```python
from build123d import *

# Parameters (mm, degrees)
SKETCH1_R            = 49.403
BOSS_EXTRUDE1_DEPTH  = 6.35
THREADED_ROD_HOLES_D = 7.9375
U_BOLT_HOLES_D       = 7.9375


with BuildPart() as part:
    # Sketch1 → Boss-Extrude1 (new body)
    with BuildSketch(Plane(origin=(0, 0, 0), x_dir=(1, 0, 0), z_dir=(0, 1, 0))):
        Circle(SKETCH1_R)
    extrude(amount=BOSS_EXTRUDE1_DEPTH)

    # Threaded Rod Holes (through all)
    with Locations(Plane(origin=(0, 6.35, 0), x_dir=(1, 0, 0), z_dir=(0, 1, 0))):
        with Locations((0, 19.05), (0, -19.05)):
            Hole(THREADED_ROD_HOLES_D / 2)

    # U-Bolt Holes (through all)
    with Locations(Plane(origin=(0, 6.35, 0), x_dir=(1, 0, 0), z_dir=(0, 1, 0))):
        with Locations((-16.66875, 0), (16.66875, 0)):
            Hole(U_BOLT_HOLES_D / 2)


solid = part.part
```
Geometry: final body of the model. Coordinates: model frame, mm. Give positions to 0.01 mm unless a question says otherwise; leave off trailing zeros. Write each loop counter-clockwise with the first axis right and the second up, starting at its lowest first coordinate (ties: lowest second). Pieces come first, ordered by that corner, then holes.
1. Section query D-D, the plane x = 19. Return loops of the section in (y, z).
2. Section query C-C, the plane y = 1.25. Return loops of the section in (x, z), then the cut area to 3 significant figures.
3. Draft query along Z for faces 1 (the cylindrical face through (-39.205, 3.131, 30.061)), 2 (the flat face through (-1, 6.35, -1)), 3 (the cylindrical face through (-20.335, 3.131, 1.52)), 4 (the cylindrical face through (0.517, 3.131, 15.115)). Return one class per face: released by +Z, released by -Z, zero draft, split by the parting line, or undercut.
4. Section query B-B, the plane z = 0. Return loops of the section in (x, y).
5. Line query: probe 1 along Z at (x, y) = (0, 2.5); probe 2 along Z at (x, y) = (1, 4.5); probe 3 along X at (y, z) = (1.75, 19.05). Output: solid intervals per line, ascending.
6. Pin query (flat end, axial travel): P1, Ø3, axis at y = 2.5, z = -0.5, coming from the -X side; P2, Ø2, axis at y = 2, z = 30, coming from the +X side. Return the tip coordinate at first contact, or that it passes through.
7. Section query A-A, the plane x = 0. Return loops of the section in (y, z), then the cut area to 3 significant figures.
Computed:
1. outline: (0, -45.6) - (6.35, -45.6) - (6.35, -3.21) - (0, -3.21) - close; (0, 3.21) - (6.35, 3.21) - (6.35, 45.6) - (0, 45.6) - close
2. outline: circle Ø98.81 at (0, 0); hole circle Ø7.94 at (-16.67, 0); hole circle Ø7.94 at (0, -19.05); hole circle Ø7.94 at (0, 19.05); hole circle Ø7.94 at (16.67, 0)
2. area: 7,470 mm2
3. face 1: split by the parting line
3. face 2: zero draft
3. face 3: undercut
3. face 4: undercut
4. outline: (-49.4, 0) - (-20.64, 0) - (-20.64, 6.35) - (-49.4, 6.35) - close; (-12.7, 0) - (12.7, 0) - (12.7, 6.35) - (-12.7, 6.35) - close; (20.64, 0) - (49.4, 0) - (49.4, 6.35) - (20.64, 6.35) - close
5. probe 1: z = -49.4 to -23.02, -15.08 to 15.08, 23.02 to 49.4
5. probe 2: z = -49.39 to -22.89, -15.21 to 15.21, 22.89 to 49.39
5. probe 3: x = -45.58 to -3.97, 3.97 to 45.58
6. P1: stops at x = -49.4
6. P2: stops at x = 40
7. outline: (0, -49.4) - (6.35, -49.4) - (6.35, -23.02) - (0, -23.02) - close; (0, -15.08) - (6.35, -15.08) - (6.35, 15.08) - (0, 15.08) - close; (0, 23.02) - (6.35, 23.02) - (6.35, 49.4) - (0, 49.4) - close
7. area: 527 mm2
